```python
from build123d import *

# Parameters (mm, degrees)
SKIZZE3_W                            = 100
SKIZZE3_H                            = 6
AUFSATZ_LINEAR_AUSTRAGEN2_DEPTH      = 70
AUFSATZ_LINEAR_AUSTRAGEN2_DEPTH_BACK = 70
HOLES_R                              = 6
HOLES_R_2                            = 3
SCHNITT_LINEAR_AUSTRAGEN2_DEPTH      = 205
SKIZZE6_R                            = 3
SCHNITT_LINEAR_AUSTRAGEN3_DEPTH      = 205


with BuildPart() as part:
    # Skizze3 → Aufsatz-Linear austragen2 (new, two sides)
    with BuildSketch(Plane(origin=(0, 0, 0), x_dir=(0, 0, -1), z_dir=(1, 0, 0))) as aufsatz_linear_austragen2_sk:
        with Locations((-82.65, 202)):
            Rectangle(SKIZZE3_W, SKIZZE3_H)
    extrude(amount=AUFSATZ_LINEAR_AUSTRAGEN2_DEPTH)
    extrude(aufsatz_linear_austragen2_sk.sketch, amount=-AUFSATZ_LINEAR_AUSTRAGEN2_DEPTH_BACK)

    # Holes → Schnitt-Linear austragen2 (cut)
    with BuildSketch(Plane(origin=(0, 0, 0), x_dir=(1, 0, 0), z_dir=(0, 1, 0))):
        with Locations(Location((0, -62.65, 0), (0, 0, 90))):
            Circle(HOLES_R)
        with Locations(Location((-40, -112.65, 0), (0, 0, 90))):
            Circle(HOLES_R_2)
        with Locations(Location((-40, -95.839319437, 0), (0, 0, 90))):
            Circle(HOLES_R_2)
        with Locations(Location((40, -95.839319437, 0), (0, 0, 90))):
            Circle(HOLES_R_2)
        with Locations(Location((40, -112.65, 0), (0, 0, 90))):
            Circle(HOLES_R_2)
    extrude(amount=SCHNITT_LINEAR_AUSTRAGEN2_DEPTH, mode=Mode.SUBTRACT)

    # Skizze6 → Schnitt-Linear austragen3 (cut)
    with BuildSketch(Plane(origin=(0, 0, 0), x_dir=(1, 0, 0), z_dir=(0, 1, 0))):
        with Locations(Location((-60, -42.65, 0), (0, 0, 90))):
            Circle(SKIZZE6_R)
        with Locations(Location((60, -42.65, 0), (0, 0, 90))):
            Circle(SKIZZE6_R)
        with Locations(Location((60, -122.65, 0), (0, 0, 90))):
            Circle(SKIZZE6_R)
        with Locations(Location((-60, -122.65, 0), (0, 0, 90))):
            Circle(SKIZZE6_R)
    extrude(amount=SCHNITT_LINEAR_AUSTRAGEN3_DEPTH, mode=Mode.SUBTRACT)


solid = part.part
```
Read the model definition and answer for the solid it produces. Units are mm, in the model's axes. Round coordinates to 2 decimals unless told otherwise and drop trailing zeros. Loops run counter-clockwise (first coordinate to the right, second up) from the corner with the lowest first, then second, coordinate; pieces in that order, holes last. Notation, with made-up numbers: (78, -8.5) -> (85, -8.5) arc R23 ccw to (85, 15.5) -> close; hole circle Ø4 at (-11.5, 70.5). An arc over 180 degrees is marked (long way). One line per item, written item: value.
1) A cutting plane is placed at B-B (x = 0). Determine the outline of the cut face in (y, z), and give its area (3 significant figures).
Answer list:
outline: (199, 32.65) -> (205, 32.65) -> (205, 56.65) -> (199, 56.65) -> close; (199, 68.65) -> (205, 68.65) -> (205, 132.65) -> (199, 132.65) -> close
area: 528 mm²
2) Consider L1, parallel to X at y = 203.6, z = 122.65; L2, parallel to Z at x = 60, y = 202.15; L3, parallel to X at y = 201.8, z = 112.65. Determine where each line is inside the solid, lowest interval first. Write a range as [from, to].
Answer list:
L1: x = [-70, -63], [-57, 57], [63, 70]
L2: z = [32.65, 39.65], [45.65, 119.65], [125.65, 132.65]
L3: x = [-70, -43], [-37, 37], [43, 70]
3) A cutting plane is placed at C-C (x = 60). Determine the outline of the cut face in (y, z), and give its area (3 significant figures).
Answer list:
outline: (199, 32.65) -> (205, 32.65) -> (205, 39.65) -> (199, 39.65) -> close; (199, 45.65) -> (205, 45.65) -> (205, 119.65) -> (199, 119.65) -> close; (199, 125.65) -> (205, 125.65) -> (205, 132.65) -> (199, 132.65) -> close
area: 528 mm²
4) A cutting plane is placed at A-A (z = 42.65). Determine the outline of the cut face in (x, y).
Answer list:
outline: (-70, 199) -> (-63, 199) -> (-63, 205) -> (-70, 205) -> close; (-57, 199) -> (57, 199) -> (57, 205) -> (-57, 205) -> close; (63, 199) -> (70, 199) -> (70, 205) -> (63, 205) -> close
5) The mould has two halves that part along X. Classify faces 1 (the face through (-70, 202, 83)), 2 (the face through (-40.132, 201.958, 98.836)), 3 (the face through (1, 202, 132.65)): pulls with the +X half, pulls with the -X half, needs draft (parallel to the pull), parting line crosses it, or undercut.
Answer list:
face 1: pulls with the -X half
face 2: undercut
face 3: needs draft
